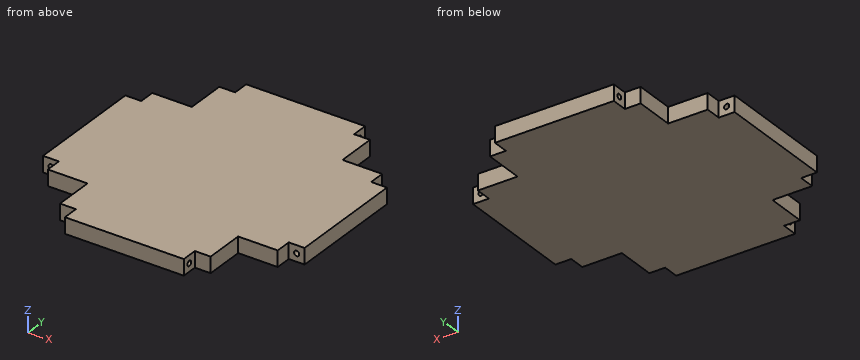
Autodesk Inventor part; units mm, degrees
ref_plane "YZ Plane" through (0, 0, 0) normal (1, 0, 0) x (0, 1, 0)
ref_plane "XZ Plane" through (0, 0, 0) normal (0, 1, 0) x (-1, 0, 0)
ref_plane "XY Plane" through (0, 0, 0) normal (0, 0, 1) x (1, 0, 0)
sketch "Sketch1" plane through (0, 0, 0) normal (0, 0, 1) x (1, 0, 0)
  line L0 (0, 82.5) -> (37.5, 82.5)
  line L1 (37.5, 82.5) -> (37.5, 72.5)
  line L2 (37.5, 72.5) -> (47.5, 72.5)
  line L3 (0, 101.1294) -> (0, 0)
  line L4 (0, 0) -> (69.4378, 0)
  line L5 (72.5, 47.5) -> (72.5, 37.5)
  line L6 (72.5, 37.5) -> (82.5, 37.5)
  line L7 (82.5, 37.5) -> (82.5, 0)
  line L8 (47.5, 72.5) -> (47.5, 47.5)
  line L9 (47.5, 47.5) -> (72.5, 47.5)
  line L10 (-82.5, 0) -> (-82.5, 37.5)
  line L11 (-82.5, 37.5) -> (-72.5, 37.5)
  line L12 (-72.5, 37.5) -> (-72.5, 47.5)
  line L13 (0, 0) -> (0, 69.4378)
  line L14 (-47.5, 72.5) -> (-37.5, 72.5)
  line L15 (-37.5, 72.5) -> (-37.5, 82.5)
  line L16 (-37.5, 82.5) -> (0, 82.5)
  line L17 (-72.5, 47.5) -> (-47.5, 47.5)
  line L18 (-47.5, 47.5) -> (-47.5, 72.5)
  line L19 (0, -82.5) -> (-37.5, -82.5)
  line L20 (-37.5, -82.5) -> (-37.5, -72.5)
  line L21 (-37.5, -72.5) -> (-47.5, -72.5)
  line L22 (0, 0) -> (-69.4378, 0)
  line L23 (-72.5, -47.5) -> (-72.5, -37.5)
  line L24 (-72.5, -37.5) -> (-82.5, -37.5)
  line L25 (-82.5, -37.5) -> (-82.5, 0)
  line L26 (-47.5, -72.5) -> (-47.5, -47.5)
  line L27 (-47.5, -47.5) -> (-72.5, -47.5)
  line L28 (82.5, 0) -> (82.5, -37.5)
  line L29 (82.5, -37.5) -> (72.5, -37.5)
  line L30 (72.5, -37.5) -> (72.5, -47.5)
  line L31 (0, 0) -> (0, -69.4378)
  line L32 (47.5, -72.5) -> (37.5, -72.5)
  line L33 (37.5, -72.5) -> (37.5, -82.5)
  line L34 (37.5, -82.5) -> (0, -82.5)
  line L35 (72.5, -47.5) -> (47.5, -47.5)
  line L36 (47.5, -47.5) -> (47.5, -72.5)
  point P0 (0, 50.5647)
  point P1 (-50.5647, 0)
  point P2 (0, -50.5647)
  point P3 (50.5647, 0)
  point P4 (82.5, 0)
  dimension "d0" = 75
  dimension "d1" = 165
  dimension "d2" = 10
  dimension "d3" = 10
  dimension "d4" = 165
  dimension "d5" = 75
  dimension "d25" = 10
  dimension "d26" = 10
  dimension "d29" = 360
extrude "Extrusion1" add sketch "Sketch1" along normal blind 10
sketch "Sketch2" plane through (37.5, 72.5, 0) normal (1, 0, 0) x (0, 0, -1)
  circle A0 centre (-5, 5) radius 2
  line L0 (0, 0) -> (0, 10)
  line L1 (0, 10) -> (-10, 10)
  point P0 (0, -72.5)
  dimension "d12" = 4
  dimension "d13" = 5
  dimension "d14" = 5
hole "Hole1" at (37.5, 77.5, 5) direction (-1, 0, 0) diameter 3.242 depth 11.8 tip angle 118
mirror "Mirror1" about plane through (0, 0, 0) normal (1, 0, 0) of "Hole1"
pattern_circular "Circular Pattern1" count 4 over 360 about axis through (0, 0, -10) along (0, 0, 1) of "Hole1", "Mirror1"
properties part number "gearbox_cap" material "PMMA Plastic"
Could you check a few things on this model? Use its own coordinates, in mm. Give positions to 0.01 mm unless a question says otherwise; leave off trailing zeros. Order: outer loops, then holes, each group sorted by start corner. A loop starts at its lowest first (then second) coordinate and runs counter-clockwise, first axis right, second up.
1. For pin 1 (1.9 mm diameter, centred on y = -77.5, z = 5, fed in from -X); pin 2 (3 mm diameter, centred on x = -77.5, z = 5, fed in from +Y); pin 3 (4 mm diameter, centred on y = -77.5, z = 5, fed in from +X), each with a flat end and sliding along its axis, tell me the tip position at first contact or that it passes through.
Answers below:
pin 1: stops at x = -25.3
pin 2: stops at y = 25.63
pin 3: stops at x = 37.5
2. Suppose I cut it at A-A (y = 68.5). Write out the boundary of the cut face in (x, z).
Answers below:
outline: (-47.5, 0) - (47.5, 0) - (47.5, 10) - (-47.5, 10) - close
3. I need wall thicknesses on L1, parallel to X at y = -31.75, z = 5; L2, parallel to Z at x = 31, y = 77.5. Which ranges of each line are inside material? Lowest first, please.
Answers below:
L1: x = -82.5 to -79.12, -75.88 to 75.88, 79.12 to 82.5
L2: z = 0 to 3.38, 6.62 to 10
4. Suppose I cut it at B-B (x = 43.5). Write out the boundary of the cut face in (y, z), plus the area to 3 significant figures.
Answers below:
outline: (-72.5, 0) - (72.5, 0) - (72.5, 10) - (-72.5, 10) - close
area: 1,450 mm2
